from build123d import *

# Parameters (mm, degrees)
SKETCH1_R           = 3.5
BOSS_EXTRUDE2_DEPTH = 1.7
FILLET1_R           = 5
FILLET2_R           = 2


with BuildPart() as part:
    # Sketch1 → Boss-Extrude2 (new body)
    with BuildSketch(Plane.XY):
        with BuildLine():
            Line((35.345416088, -38.173843213), (16.206796624, -19.035223749))
            ThreePointArc((16.206796624, -19.035223749), (0, -25), (-16.206796624, -19.035223749))
            Line((-16.206796624, -19.035223749), (-35.345416088, -38.173843213))
            ThreePointArc((-35.345416088, -38.173843213), (-43.535533906, -43.535533906), (-38.173843213, -35.345416088))
            Line((-38.173843213, -35.345416088), (-19.035223749, -16.206796624))
            ThreePointArc((-19.035223749, -16.206796624), (-25, 0), (-19.035223749, 16.206796624))
            Line((-19.035223749, 16.206796624), (-38.173843213, 35.345416088))
            ThreePointArc((-38.173843213, 35.345416088), (-43.535533906, 43.535533906), (-35.345416088, 38.173843213))
            Line((-35.345416088, 38.173843213), (-16.206796624, 19.035223749))
            ThreePointArc((-16.206796624, 19.035223749), (0, 25), (16.206796624, 19.035223749))
            Line((16.206796624, 19.035223749), (35.345416088, 38.173843213))
            ThreePointArc((35.345416088, 38.173843213), (43.535533906, 43.535533906), (38.173843213, 35.345416088))
            Line((38.173843213, 35.345416088), (19.035223749, 16.206796624))
            ThreePointArc((19.035223749, 16.206796624), (25, 0), (19.035223749, -16.206796624))
            Line((19.035223749, -16.206796624), (38.173843213, -35.345416088))
            ThreePointArc((38.173843213, -35.345416088), (43.535533906, -43.535533906), (35.345416088, -38.173843213))
        make_face()
        with Locations((-40, 40)):
            Circle(SKETCH1_R, mode=Mode.SUBTRACT)
        with Locations((40, 40)):
            Circle(SKETCH1_R, mode=Mode.SUBTRACT)
        with Locations((40, -40)):
            Circle(SKETCH1_R, mode=Mode.SUBTRACT)
        with Locations((-40, -40)):
            Circle(SKETCH1_R, mode=Mode.SUBTRACT)
    extrude(amount=BOSS_EXTRUDE2_DEPTH)

    # Fillet1
    fillet1_edges = [part.edges().sort_by_distance(p)[0] for p in [
        (16.206796624, 19.035223749, 0.85),
        (19.035223749, 16.206796624, 0.85),
        (19.035223749, -16.206796624, 0.85),
        (16.206796624, -19.035223749, 0.85),
        (-16.206796624, -19.035223749, 0.85),
        (-19.035223749, -16.206796624, 0.85),
        (-19.035223749, 16.206796624, 0.85),
        (-16.206796624, 19.035223749, 0.85),
    ]]
    fillet(fillet1_edges, radius=FILLET1_R)

    # Fillet2
    fillet2_edges = [part.edges().sort_by_distance(p)[0] for p in [
        (35.345416088, 38.173843213, 0.85),
        (38.173843213, 35.345416088, 0.85),
        (38.173843213, -35.345416088, 0.85),
        (35.345416088, -38.173843213, 0.85),
        (-35.345416088, -38.173843213, 0.85),
        (-38.173843213, -35.345416088, 0.85),
        (-38.173843213, 35.345416088, 0.85),
        (-35.345416088, 38.173843213, 0.85),
    ]]
    fillet(fillet2_edges, radius=FILLET2_R)


solid = part.part
CAD build for the part. Positions are in the model's coordinates, mm. A direction names the side the tool comes from. Round coordinates to 2 decimals unless told otherwise and drop trailing zeros. Order: outer loops, then holes, each group sorted by start corner. A loop starts at its lowest first (then second) coordinate and runs counter-clockwise, first axis right, second up. Notation, with made-up numbers: (61, 86.5) -> (108, 86.5) arc R25 ccw to (108, 119.5) -> close; hole circle Ø8 at (66.5, 82.25). An arc over 180 degrees is marked (long way). Write item = value, one per line. Start each with the question number.
(1) Which spindle directions (+Z, -Z, +X, -X, +Y, -Y) get a long thin tool onto all of the face, cutting with end or side? Do faces 5 (the flat face through (26.976, -29.804, 0.838)), 6 (the flat face through (-29.804, -26.976, 0.838)), 7 (the flat face through (-26.976, 29.804, 0.838)). Say none if no direction does.
(2) Cut at D-D, the plane z = 1.35. State how many separate pieces and enclosed holes the cut face has, then the cut area to 3 significant figures.
(3) Pull direction X, two halves, no side cores. Call faces 1 (the cylindrical face through (-25, 0, 1)), 2 (the flat face through (0, 4, 1.7)), 3 (the cylindrical face through (-42.58, -37.635, 0.838)), 4 (the cylindrical face through (-44, 43, 1)): released by +X, released by -X, zero draft, split by the parting line, or undercut.
(4) Probe line 1 (Y direction, x = -40, z = 1.2); line 2 (X direction, y = -21, z = 1.55); line 3 (X direction, y = 38, z = 1.55). List the from-to ranges inside material, lowest first. Write a range as [from, to].
(5) Cut at C-C, the plane y = 7. List the corners of the cut face in (x, z), then the cut area to 3 significant figures.
(6) Pin check, flat tip, straight feed: P1, Ø4, axis at x = 29, y = 22, coming from the -Z side. Stop position of the tip, or through.
(7) Cut at A-A, the plane y = 33. List the corners of the cut face in (x, z).
Model answer:
q1.face_5 = +Z, -Z, -Y
q1.face_6 = +Z, -Z, -X
q1.face_7 = +Z, -Z, +Y
q2.separate_pieces = 1
q2.enclosed_holes = 4
q2.area = 2,580 mm2
q3.face_1 = released by -X
q3.face_2 = zero draft
q3.face_3 = undercut
q3.face_4 = undercut
q4.line_1 = [-45, -43.5], [-36.5, -35], [35, 36.5], [43.5, 45]
q4.line_2 = [-23.83, -17.69], [-13.67, 13.67], [17.69, 23.83]
q4.line_3 = [-44.58, -42.87], [-37.13, -34.96], [34.96, 37.13], [42.87, 44.58]
q5.outline = (-24, 0) -> (24, 0) -> (24, 1.7) -> (-24, 1.7) -> close
q5.area = 81.6 mm2
q6.P1 = through
q7.outline = (-35.83, 0) -> (-30.17, 0) -> (-30.17, 1.7) -> (-35.83, 1.7) -> close; (30.17, 0) -> (35.83, 0) -> (35.83, 1.7) -> (30.17, 1.7) -> close
